Source: CAD feature listing. Evaluate the final solid. Frame: model axes, mm. A direction names the side the tool comes from. Round coordinates to 2 decimals unless told otherwise and drop trailing zeros. Loops run counter-clockwise (first coordinate to the right, second up) from the corner with the lowest first, then second, coordinate; pieces in that order, holes last. Notation, with made-up numbers: M 54,85.25 L 92,85.25 A13 cw 92,89.25 Z; hole C 78,73 d7. An arc over 180 degrees is marked long. One line per item, written item: value.
from build123d import *

# Parameters (mm, degrees)
EXTRU_MINCE1_DEPTH = 100
EXTRUSION2_DEPTH   = 2


with BuildPart() as part:
    # Esquisse1 → Extru.-Mince1 (new body)
    with BuildSketch(Plane.XY):
        Polygon((-49.585494923, -0.363286713), (-28.372291487, 36.379059428), (3.108706941, 36.379059428), (28.083525041, 79.636713287), (150.414505077, 79.636713287), (150.414505077, -0.363286713), (148.414505077, -0.363286713), (148.414505077, 77.636713287), (29.238225579, 77.636713287), (4.263407479, 34.379059428), (-27.217590949, 34.379059428), (-47.853444115, -1.363286713), align=None)
    extrude(amount=EXTRU_MINCE1_DEPTH)

    # Esquisse2 → Extrusion2 (add)
    with BuildSketch(Plane.XY.offset(100)):
        Polygon((27.911407902, -1.363286713), (-47.853444115, -1.363286713), (-49.585494923, -0.363286713), (-28.372291487, 36.379059428), (3.108706941, 36.379059428), (27.899141653, 79.636713287), (150.414505077, 79.636713287), (150.414505077, -1.363286713), align=None)
    extrude(amount=EXTRUSION2_DEPTH)


solid = part.part
1. Section query B-B (x = 46). Return the cut outline in (y, z), and give its area (3 significant figures).
Report:
outline: M -1.36,100 L 77.64,100 L 77.64,0 L 79.64,0 L 79.64,102 L -1.36,102 Z
area: 362 mm2
2. Ray query, line 1 (Z direction, x = 19.5, y = 35); line 2 (Y direction, x = 66, z = 6); line 3 (Y direction, x = -7, z = 61). Return the intervals inside material, ascending. Write a range as [from, to].
Report:
line 1: z = [100, 102]
line 2: y = [77.64, 79.64]
line 3: y = [34.38, 36.38]
3. Pin query (flat end, axial travel): pin 1 (3 mm diameter, centred on x = 3.5, z = 76.5, fed in from +Y); pin 2 (2 mm diameter, centred on x = 99.5, z = 27.5, fed in from -Y); pin 3 (9.5 mm diameter, centred on x = -4, z = 70.5, fed in from -Y). Return the tip coordinate at first contact, or that it passes through.
Report:
pin 1: stops at y = 39.65
pin 2: stops at y = 77.64
pin 3: stops at y = 34.38
4. Pull-direction query (X, two-part tool) for faces 5 (the face through (74, 40, 102)), 6 (the face through (-39.1, 17.8, 50.3)), 7 (the face through (-37.39, 16.76, 49.3)); classes: released by +X, released by -X, zero draft, split by the parting line, or undercut.
Report:
face 5: zero draft
face 6: released by -X
face 7: undercut
5. Section query D-D (x = -12). Return the cut outline in (y, z).
Report:
outline: M -1.36,100 L 34.38,100 L 34.38,0 L 36.38,0 L 36.38,102 L -1.36,102 Z
6. Section query C-C (y = 67). Return the cut outline in (x, z), and give its area (3 significant figures).
Report:
outline: M 20.66,100 L 20.79,100 L 20.79,0 L 23.1,0 L 23.1,100 L 148.41,100 L 148.41,0 L 150.41,0 L 150.41,102 L 20.66,102 Z
area: 690 mm2
7. Reachability of faces 1 (the face through (-11, 34.379, 49)), 2 (the face through (88, 79.637, 50)), 3 (the face through (15.421, 57.705, 49.3)), 4 (the face through (-13, 36.379, 50)) from +Z, -Z, +X, -X, +Y, -Y: full face, straight path, thin tool, end or side. Return the list, or none.
Report:
face 1: -Z, -Y
face 2: +Z, -Z, +X, -X, +Y
face 3: -Z, -X, +Y
face 4: +Z, -Z, -X, +Y
8. Section query A-A (z = 94). Return the cut outline in (x, y).
Report:
outline: M -49.59,-0.36 L -47.85,-1.36 L -27.22,34.38 L 4.26,34.38 L 29.24,77.64 L 148.41,77.64 L 148.41,-0.36 L 150.41,-0.36 L 150.41,79.64 L 28.08,79.64 L 3.11,36.38 L -28.37,36.38 Z
